from build123d import *

# Parameters (mm, degrees)
BOSS_EXTRUDE1_DEPTH     = 38.1
CUT_EXTRUDE1_DEPTH      = 43.337483392
CUT_EXTRUDE1_DEPTH_BACK = 43.337483392
SKETCH2_R               = 2.07
CHAMFER1_SIZE           = 2
FILLET1_R               = 2


with BuildPart() as part:
    # Sketch1 → Boss-Extrude1 (new, symmetric)
    with BuildSketch(Plane.XY):
        Polygon((-17.7, -7.7), (-17.7, -17.7), (17.7, -17.7), (17.7, -7.7), (12.95, -7.7), (12.95, -12.95), (-12.95, -12.95), (-12.95, -7.7), align=None)
    extrude(amount=BOSS_EXTRUDE1_DEPTH, both=True)

    # Sketch2 → Cut-Extrude1 (cut, two sides: drawn at the far end of the back side and taken through both)
    with BuildSketch(Plane(origin=(0, -12.95, 0), x_dir=(1, 0, 0), z_dir=(0, 1, 0)).offset(-CUT_EXTRUDE1_DEPTH_BACK)):
        with Locations(Location((0, 25.4, 0), (0, 0, 270))):
            Circle(SKETCH2_R)
        with Locations(Location((0, 12.7, 0), (0, 0, 270))):
            Circle(SKETCH2_R)
        with Locations(Location((0, 0, 0), (0, 0, 270))):
            Circle(SKETCH2_R)
        with Locations(Location((0, -12.7, 0), (0, 0, 270))):
            Circle(SKETCH2_R)
        with Locations(Location((0, -25.4, 0), (0, 0, 270))):
            Circle(SKETCH2_R)
        with Locations((0, -38.1)):
            Circle(SKETCH2_R)
        with Locations((0, 38.1)):
            Circle(SKETCH2_R)
    extrude(amount=CUT_EXTRUDE1_DEPTH + CUT_EXTRUDE1_DEPTH_BACK, mode=Mode.SUBTRACT)

    # Chamfer1
    chamfer1_edges = [part.edges().sort_by_distance(p)[0] for p in [
        (-12.95, -7.7, 0),
        (12.95, -7.7, 0),
    ]]
    chamfer(chamfer1_edges, length=CHAMFER1_SIZE)

    # Fillet1
    fillet1_edges = [part.edges().sort_by_distance(p)[0] for p in [
        (-17.7, -17.7, 0),
        (-17.7, -7.7, 0),
        (17.7, -7.7, 0),
        (17.7, -17.7, 0),
    ]]
    fillet(fillet1_edges, radius=FILLET1_R)


solid = part.part
Geometry check sheet. Reference: the model listing, model coordinates, mm. A direction names the side the tool comes from. Coordinates: 2 decimals unless noted, no trailing zeros. Write each loop counter-clockwise with the first axis right and the second up, starting at its lowest first coordinate (ties: lowest second). Pieces come first, ordered by that corner, then holes. Notation, with made-up numbers: (15.5, 14.25) -> (59.5, 14.25) arc R4 ccw to (59.5, 18.25) -> close; hole circle Ø2 at (77.5, 36.25). An arc over 180 degrees is marked (long way). One line per question, with ' | ' between items.
1. Cross-section at A-A on x = 0. Record the cut outline in (y, z), and give its area (3 significant figures).
Answers:
outline: (-17.7, -36.03) -> (-12.95, -36.03) -> (-12.95, -27.47) -> (-17.7, -27.47) -> close; (-17.7, -23.33) -> (-12.95, -23.33) -> (-12.95, -14.77) -> (-17.7, -14.77) -> close; (-17.7, -10.63) -> (-12.95, -10.63) -> (-12.95, -2.07) -> (-17.7, -2.07) -> close; (-17.7, 2.07) -> (-12.95, 2.07) -> (-12.95, 10.63) -> (-17.7, 10.63) -> close; (-17.7, 14.77) -> (-12.95, 14.77) -> (-12.95, 23.33) -> (-17.7, 23.33) -> close; (-17.7, 27.47) -> (-12.95, 27.47) -> (-12.95, 36.03) -> (-17.7, 36.03) -> close | area: 244 mm²
2. Cross-section at D-D on y = -13.75. Record the cut outline in (x, z).
Answers:
outline: (-17.7, -38.1) -> (-2.07, -38.1) arc R2.07 cw to (2.07, -38.1) -> (17.7, -38.1) -> (17.7, 38.1) -> (2.07, 38.1) arc R2.07 cw to (-2.07, 38.1) -> (-17.7, 38.1) -> close; hole circle Ø4.14 at (0, -25.4); hole circle Ø4.14 at (0, -12.7); hole circle Ø4.14 at (0, 0); hole circle Ø4.14 at (0, 12.7); hole circle Ø4.14 at (0, 25.4)
3. Cross-section at B-B on z = 0. Record the cut outline in (x, y), and give its area (3 significant figures).
Answers:
outline: (-17.7, -15.7) arc R2 ccw to (-15.7, -17.7) -> (-2.07, -17.7) -> (-2.07, -12.95) -> (-12.95, -12.95) -> (-12.95, -9.7) -> (-14.95, -7.7) -> (-15.7, -7.7) arc R2 ccw to (-17.7, -9.7) -> close; (2.07, -17.7) -> (15.7, -17.7) arc R2 ccw to (17.7, -15.7) -> (17.7, -9.7) arc R2 ccw to (15.7, -7.7) -> (14.95, -7.7) -> (12.95, -9.7) -> (12.95, -12.95) -> (2.07, -12.95) -> close | area: 191 mm²
4. Draft check along Z on faces 1 (the flat face through (12, -14, 38.1)), 2 (the cylindrical face through (0.09, -15.36, -14.77)), 3 (the flat face through (13.96, -8.69, -0.53)). Enter one of: +Z half, -Z half, draft (parallel to the pull), parting line (faces both ways), or undercut.
Answers:
face 1: +Z half | face 2: undercut | face 3: draft
5. Set-up check for faces 4 (the flat face through (-12.95, -11, 1)), 5 (the flat face through (-12, -14, 38.1)): record each of +Z, -Z, +X, -X, +Y, -Y from which the full face is reachable in a straight line by a thin tool's end or side.
Answers:
face 4: +Z, -Z, +Y | face 5: +Z, +X, -X, +Y, -Y
6. Thickness scan on probe 1 along Z at (x, y) = (0, -14); probe 2 along X at (y, z) = (-11.5, -12). Record the ranges inside material, lowest first. Write a range as from..to.
Answers:
probe 1: z = -36.03..-27.47, -23.33..-14.77, -10.63..-2.07, 2.07..10.63, 14.77..23.33, 27.47..36.03 | probe 2: x = -17.7..-12.95, 12.95..17.7
7. Cross-section at C-C on y = -8.5. Record the cut outline in (x, z).
Answers:
outline: (-17.3, -38.1) -> (-14.15, -38.1) -> (-14.15, 38.1) -> (-17.3, 38.1) -> close; (14.15, -38.1) -> (17.3, -38.1) -> (17.3, 38.1) -> (14.15, 38.1) -> close
8. Depth check by flat-ended pin: pin 1 Ø8 at (x, z) = (-2.5, -4) entering from +Y; pin 2 Ø3.5 at (x, z) = (0, -25.4) entering from -Y; pin 3 Ø3 at (x, z) = (-12.5, -11.5) entering from +Y; pin 4 Ø1.5 at (x, z) = (-12.5, 22) entering from +Y. Enter the tip coordinate at first touch or a pass-through.
Answers:
pin 1: stops at y = -12.95 | pin 2: passes through | pin 3: stops at y = -8.65 | pin 4: stops at y = -9.4
